Can you work these out from the model? Positions are in its coordinate system, mm. Face numbers are marked on the shaded views. Coordinates: 2 decimals unless noted, no trailing zeros. Order: outer loops, then holes, each group sorted by start corner. A loop starts at its lowest first (then second) coordinate and runs counter-clockwise, first axis right, second up.
```python
from build123d import *

# Parameters (mm, degrees)
F1_DEPTH = 2.794
F2_W     = 368.3
F2_H     = 139.9649612151
F3_DEPTH = 0.762
F4_W     = 175.4610008955
F4_H     = 70.8550387849
F5_DEPTH = 1.27
F6_W     = 15.326482141
F6_H     = 14.1157105111
F7_DEPTH = 0.508


with BuildPart() as f1:
    # F0 (on Top) → F1 (new body)
    with BuildSketch(Plane.XY):
        with BuildLine():
            ThreePointArc((191.6694995522, 125.0495699547), (189.8096276128, 129.5396980153), (185.3194995522, 131.3995699547))
            Line((185.3194995522, 131.3995699547), (-195.6805004478, 131.3995699547))
            ThreePointArc((-195.6805004478, 131.3995699547), (-200.1706285083, 129.5396980153), (-202.0305004478, 125.0495699547))
            Line((-202.0305004478, 125.0495699547), (-202.0305004478, -111.1704300453))
            ThreePointArc((-202.0305004478, -111.1704300453), (-200.1706285083, -115.6605581058), (-195.6805004478, -117.5204300453))
            Line((-195.6805004478, -117.5204300453), (185.3194995522, -117.5204300453))
            ThreePointArc((185.3194995522, -117.5204300453), (189.8096276128, -115.6605581058), (191.6694995522, -111.1704300453))
            Line((191.6694995522, -111.1704300453), (191.6694995522, 125.0495699547))
        make_face()
    extrude(amount=F1_DEPTH)

    # F2 (on face) → F3 (cut)
    with BuildSketch(Plane.XY.offset(2.794)):
        with Locations((-5.1805004478, 48.7170893472)):
            Rectangle(F2_W, F2_H)
    extrude(amount=-F3_DEPTH, mode=Mode.SUBTRACT)

    # F4 (on face) → F5 (cut)
    with BuildSketch(Plane.XY.offset(2.794)):
        with Locations((0, -71.9329106528)):
            Rectangle(F4_W, F4_H)
    extrude(amount=-F5_DEPTH, mode=Mode.SUBTRACT)

    # F6 (on face) → F7 (join)
    with BuildSketch(Plane.XY.offset(2.032)):
        with Locations((-181.6672593772, 111.6417146992)):
            Rectangle(F6_W, F6_H)
        with Locations((-156.2672593772, 111.6417146992)):
            Rectangle(F6_W, F6_H)
        with Locations((-130.8672593772, 111.6417146992)):
            Rectangle(F6_W, F6_H)
    extrude(amount=F7_DEPTH)


solid = f1.part
```
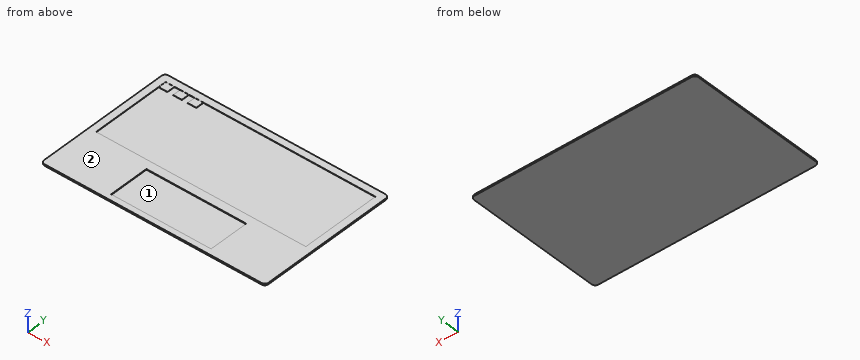
1. Please list where these lines run through material, in increasing order: probe 1 along Y at (x, z) = (-7.5, 2.35); probe 2 along X at (y, z) = (-81, 2.45); probe 3 along Y at (x, z) = (169.5, 2.15).
Completed:
probe 1: y = -117.52 to -107.36, -36.51 to -21.27, 118.7 to 131.4
probe 2: x = -202.03 to -87.73, 87.73 to 191.67
probe 3: y = -117.52 to -21.27, 118.7 to 131.4
2. Imagine slicing it at A-A on x = 124. Please give me the cut outline in (y, z).
Completed:
outline: (-117.52, 0) - (131.4, 0) - (131.4, 2.79) - (118.7, 2.79) - (118.7, 2.03) - (-21.27, 2.03) - (-21.27, 2.79) - (-117.52, 2.79) - close
3. I'm going to push flat-ended pins straight in: pin 1 (10 mm diameter, centred on x = 128.5, y = -6.5, fed in from +Z); pin 2 (2 mm diameter, centred on x = -42.5, y = -39.5, fed in from +Z); pin 3 (4 mm diameter, centred on x = -181, y = 113.5, fed in from +Z). Where does each tip first touch, or does it pass through?
Completed:
pin 1: stops at z = 2.03
pin 2: stops at z = 1.52
pin 3: stops at z = 2.54
4. Imagine slicing it at B-B on y = -51. Please give me the cut outline in (x, z).
Completed:
outline: (-202.03, 0) - (191.67, 0) - (191.67, 2.79) - (87.73, 2.79) - (87.73, 1.52) - (-87.73, 1.52) - (-87.73, 2.79) - (-202.03, 2.79) - close
5. Thinking about a two-plate mould opening in X: for the marked faces 1 and 2, which applies, pulls with the +X half, pulls with the -X half, needs draft (parallel to the pull), parting line crosses it, or undercut?
Completed:
face 1: undercut
face 2: needs draft
6. Imagine slicing it at C-C on x = -67. Please give me the cut outline in (y, z).
Completed:
outline: (-117.52, 0) - (131.4, 0) - (131.4, 2.79) - (118.7, 2.79) - (118.7, 2.03) - (-21.27, 2.03) - (-21.27, 2.79) - (-36.51, 2.79) - (-36.51, 1.52) - (-107.36, 1.52) - (-107.36, 2.79) - (-117.52, 2.79) - close
